Source: CAD feature listing. Evaluate the final solid. Frame: model axes, mm. A direction names the side the tool comes from. Round coordinates to 2 decimals unless told otherwise and drop trailing zeros. Write each loop counter-clockwise with the first axis right and the second up, starting at its lowest first coordinate (ties: lowest second). Pieces come first, ordered by that corner, then holes. Notation, with made-up numbers: M -14,-25.75 L 35,-25.75 A16 ccw 35,-20.75 Z; hole C 87,15.25 d9. An arc over 180 degrees is marked long. Answer in a Markdown table with one row per item.
Autodesk Inventor part; units mm, degrees
ref_plane "Work Plane2" through (3.35, 0, 0) normal (0, 0, -1) x (1, 0, 0)
ref_plane "YZ Plane" through (0, 0, 0) normal (1, 0, 0) x (0, 1, 0)
ref_plane "XZ Plane" through (0, 0, 0) normal (0, 1, 0) x (-1, 0, 0)
sketch "Sketch1" plane through (0, 0, 0) normal (0, 0, 1) x (1, 0, 0)
  line L0 (1.2, 0) -> (6, 0)
  line L1 (6, 0) -> (6, 1)
  line L2 (6, 1) -> (2, 1)
  line L3 (2, 1) -> (1.7546, 0.8773)
  line L4 (1.7546, 0.8773) -> (1.2, 0.8773)
  line L5 (0, 1.9) -> (0, 0.95)
  line L6 (0, 0.95) -> (0.9455, 0.4786)
  line L7 (0.9455, 0.4786) -> (1.2, 0)
  line L8 (-1.2, 0) -> (7.2, 0)
  line L9 (0, -0.38) -> (0, 2.28)
  line L10 (0, 1.9) -> (0.1773, 1.9)
  line L11 (0.1773, 1.9) -> (1.2, 0.8773)
  line L12 (2, 1) -> (1.0773, 1) construction
  dimension "d1" = 4
  dimension "d2" = 2
  dimension "d3" = 1.7546
  dimension "d4" = 1.9
  dimension "d5" = 26.5
  dimension "d6" = 62
  dimension "d7" = 1.2
  dimension "d8" = 0.2454
  dimension "d12" = 3.8
  dimension "d13" = 45
  dimension "d15" = 6
  dimension "d24" = 1.2
revolve "Body" add sketch "Sketch1" angle 360 about axis through (1.2, 0, 0) along (1, 0, 0) contours L7 L6 L5 L10 L11 L4 L3 L2 L1 L0
sketch "Sketch2" plane through (0, 0, 0) normal (-1, 0, 0) x (0, 0, 1)
  line L0 (0, 0.95) -> (0, 0) construction
  line L1 (0, 0) -> (0.95, 0) construction
  arc A0 (0.285, 0) -> (0, 0.285) centre (0, 0) ccw construction
  arc A1 (0.3325, 0) -> (0, 0.3325) centre (0, 0) ccw construction
  arc A2 (0.9373, 0.155) -> (0.155, 0.9373) centre (0, 0) ccw
  line L2 (0, 0) -> (0.6718, 0.6718) construction
  line L3 (0.155, 0.9373) -> (0.1646, 0.2889)
  line L4 (0.9373, 0.155) -> (0.2889, 0.1646)
  arc A3 (0.155, 0.9373) -> (0, 0.95) centre (0, 0) ccw
  arc A4 (0.95, 0) -> (0.9373, 0.155) centre (0, 0) ccw
  line L5 (0, -2.66) -> (0, 2.66)
  line L6 (-2.66, 0) -> (2.66, 0)
  arc A5 (0.155, -0.9373) -> (0.9373, -0.155) centre (0, 0) ccw
  line L7 (0.155, -0.9373) -> (0.1646, -0.2889)
  line L8 (0.9373, -0.155) -> (0.2889, -0.1646)
  arc A6 (0, -0.95) -> (0.155, -0.9373) centre (0, 0) ccw
  arc A7 (0.9373, -0.155) -> (0.95, 0) centre (0, 0) ccw
  arc A8 (-0.155, 0.9373) -> (-0.9373, 0.155) centre (0, 0) ccw
  line L9 (-0.155, 0.9373) -> (-0.1646, 0.2889)
  line L10 (-0.9373, 0.155) -> (-0.2889, 0.1646)
  arc A9 (0, 0.95) -> (-0.155, 0.9373) centre (0, 0) ccw
  arc A10 (-0.9373, 0.155) -> (-0.95, 0) centre (0, 0) ccw
  arc A11 (-0.155, -0.9373) -> (0, -0.95) centre (0, 0) ccw
  arc A12 (-0.9373, -0.155) -> (-0.155, -0.9373) centre (0, 0) ccw
  arc A13 (-0.95, 0) -> (-0.9373, -0.155) centre (0, 0) ccw
  line L11 (-0.9373, -0.155) -> (-0.2889, -0.1646)
  line L12 (-0.155, -0.9373) -> (-0.1646, -0.2889)
  arc A14 (0.1646, 0.2889) -> (0.2889, 0.1646) centre (0.2908, 0.2908) ccw
  arc A15 (0.2889, -0.1646) -> (0.1646, -0.2889) centre (0.2908, -0.2908) ccw
  arc A16 (-0.2889, 0.1646) -> (-0.1646, 0.2889) centre (-0.2908, 0.2908) ccw
  arc A17 (-0.1646, -0.2889) -> (-0.2889, -0.1646) centre (-0.2908, -0.2908) ccw
  point P0 (0.6718, -0.6718)
  point P1 (-0.6718, 0.6718)
  point P2 (-0.6718, -0.6718)
  dimension "d17" = 0.57
  dimension "d18" = 0.665
  dimension "d19" = 1.9
  dimension "d20" = 45
  dimension "d21" = 0.155
extrude "Slot" add sketch "Sketch2" against normal up to next draft 5 contours L4 A14 L3 A2 | A5 L7 A15 L8 | L9 A16 L10 A8 | A12 L11 A17 L12
fillet "Fillet1" radius 0.062 4 edges at (0, 0.95, 0) (0, 0, -0.95) (0, -0.95, 0) (0, 0, 0.95)
thread "Thread"
chamfer "Chamfer1" distance 0.2454 distance2 0.1227 1 edges at (6, -1, 0) measured on face at (6, 0.3275, -0.4215)
ref_plane "Work Plane2" through (3.35, 0, 0) normal (0, 0, -1) x (1, 0, 0)
equation "\"d1\" = GEL"
equation "\"d2\" = GD"
equation "\"d3\" = BDM"
equation "\"d4\" = SDM"
equation "\"d7\" = INTI"
equation "\"d8\" = GAL"
equation "\"d12\" = KOD"
equation "\"d13\" = 0.5 * SEWI"
equation "\"d15\" = NLG"
equation "\"d24\" = KOH"
equation "\"d17\" = 0.3 * SDM"
equation "\"d18\" = 0.35 * SDM"
equation "\"d19\" = SDM"
equation "\"d21\" = 0.5 * SBR"
equation "\"d23\" = 0.2 * SBR"
equation "\"d10\" = GEL"
equation "\"d25\" = -0.5 * SPD + 0.5 * GD"
equation "\"d26\" = 0.5 * GAL"
equation "\"NLG\" = 6"
equation "\"GEL\" = 4"
equation "\"GAL\" = 0.61345 * PTC"
equation "\"SPD\" = NND - 1.2269 * PTC"
equation "\"KOD\" = 3.8"
equation "\"KOH\" = 1.2"
equation "\"SBR\" = 0.31"
equation "\"INTI\" = 1.2"
equation "\"SDM\" = 1.9"
equation "\"GD\" = NND"
equation "\"BDM\" = NND - GAL"
equation "\"SEWI\" = 90deg"
equation "\"d9\" = SDM"
equation "\"GUL\" = 0.61345 * PTC"
equation "\"TOA\" = 30deg"
equation "\"EPV\" = 2.2"
equation "\"THREADDIA\" = 2"
equation "\"PTC\" = 0.4"
equation "\"NND\" = 2"
equation "\"GD1\" = THREADDIA - 1.2269 * PTC"
properties part number "ISO 7046-1 - M2 x 6 - 4.8 - H" material "Steel"
Q1. Access query for faces 1 (the flat face through (0, 0.4, -0.4)), 2 (the cylindrical face through (1.47, 0.47, -0.74)). Directions: +Z, -Z, +X, -X, +Y, -Y. A direction counts if a zero-diameter tool reaches every point of the face in a straight line with its end or side. Return the directions, or none.
Solutions:
| item | result |
|---|---|
| face 1 | +Z, -Z, -X, +Y, -Y |
| face 2 | none |
Q2. Section A-A (x = 2.5). Return loops of the section in (y, z), and give its area (3 significant figures).
Solutions:
| item | result |
|---|---|
| outline | C 0,0 d2 |
| area | 3.14 mm2 |
Q3. Contact query for flat-ended pins moving along their axis: pin 1 Ø1 at (x, z) = (2.5, -0.5) entering from +Y; pin 2 Ø1 at (x, y) = (2, 0) entering from -Z; pin 3 Ø1.5 at (x, y) = (3.5, -0.5) entering from +Z; pin 4 Ø1 at (y, z) = (-0.5, 1) entering from +X. Output: stop coordinate, or through.
Solutions:
| item | result |
|---|---|
| pin 1 | stops at y = 1 |
| pin 2 | stops at z = -1 |
| pin 3 | stops at z = 1 |
| pin 4 | stops at x = 6 |
Q4. Pull-direction query (Z, two-part tool) for faces 3 (the cylindrical face through (4, 0, 1)), 4 (the conical face through (1.2, 0, 0)), 5 (the flat face through (6, 0, 0)); classes: pulls with the +Z half, pulls with the -Z half, needs draft (parallel to the pull), parting line crosses it, or undercut.
Solutions:
| item | result |
|---|---|
| face 3 | parting line crosses it |
| face 4 | undercut |
| face 5 | needs draft |
Q5. Material intervals for probe 1 along X at (y, z) = (-1, -0.4); probe 2 along Y at (x, z) = (5.75, -0.15); probe 3 along X at (y, z) = (1.5, 0.6), sorted ascending.
Solutions:
| item | result |
|---|---|
| probe 1 | x = 0 to 1 |
| probe 2 | y = -0.99 to 0.99 |
| probe 3 | x = 0 to 0.46 |
